For this review, take the finished solid that the model builds, in its own axes (mm). A direction names the side the tool comes from. Round coordinates to 2 decimals unless told otherwise and drop trailing zeros. Write each loop counter-clockwise with the first axis right and the second up, starting at its lowest first coordinate (ties: lowest second). Pieces come first, ordered by that corner, then holes. Notation, with made-up numbers: (-22, 88) - (19, 88) arc R17 cw to (19, 96) - close; hole circle Ø3 at (-31.75, 37). An arc over 180 degrees is marked (long way). Answer in a Markdown table with one row per item. Add a question column.
from build123d import *

# Parameters (mm, degrees)
SKETCH_1_R          = 29
EXTRUDE_1_DEPTH     = 6
SKETCH_2_R          = 12
EXTRUDE_2_DEPTH     = 20
SKETCH_3_R          = 2
CUT_EXTRUDE_1_DEPTH = 10
SKETCH_4_R          = 3
CUT_EXTRUDE_2_DEPTH = 30


with BuildPart() as part:
    # 草图1 → 凸台-拉伸1 (new body)
    with BuildSketch(Plane.XY):
        Circle(SKETCH_1_R)
    extrude(amount=EXTRUDE_1_DEPTH)

    # 草图2 → 凸台-拉伸2 (add)
    with BuildSketch(Plane.XY.offset(6)):
        Circle(SKETCH_2_R)
    extrude(amount=EXTRUDE_2_DEPTH)

    # 草图3 → 切除-拉伸1 (cut)
    with BuildSketch(Plane.XY.offset(6)):
        with Locations((0, 24)):
            Circle(SKETCH_3_R)
        with Locations((20.784609691, 12)):
            Circle(SKETCH_3_R)
        with Locations((20.784609691, -12)):
            Circle(SKETCH_3_R)
        with Locations((0, -24)):
            Circle(SKETCH_3_R)
        with Locations((-20.784609691, -12)):
            Circle(SKETCH_3_R)
        with Locations((-20.784609691, 12)):
            Circle(SKETCH_3_R)
    extrude(amount=-CUT_EXTRUDE_1_DEPTH, mode=Mode.SUBTRACT)

    # 草图4 → 切除-拉伸2 (cut)
    with BuildSketch(Plane.XY.offset(26)):
        Circle(SKETCH_4_R)
    extrude(amount=-CUT_EXTRUDE_2_DEPTH, mode=Mode.SUBTRACT)


solid = part.part
Q1. Insertion check: pin 1 Ø1 at (y, z) = (14.5, 5) entering from +X; pin 2 Ø7 at (x, y) = (0, 0) entering from +Z; pin 3 Ø2 at (x, z) = (7.5, 3.5) entering from -Y; pin 4 Ø3 at (x, y) = (-20.5, 15) entering from +Z. Each pin has a flat end and moves straight along its axis. Give the tip position at first contact, or say it passes through.
Q2. To check wall thickness, follow probe 1 along Y at (x, z) = (0, 18); probe 2 along Z at (x, y) = (-22.5, -17); probe 3 along Y at (x, z) = (-1, 15). State the ranges of each line that lie inside material, in increasing order.
Q3. Add section A-A on x = 0. State the section outline as (y, z) points, then the cut area to 3 significant figures.
Q4. Add section C-C on z = 16.5. State the section outline as (x, y) points, then the cut area to 3 significant figures.
Q5. Add section B-B on y = 0. State the section outline as (x, z) points, then the cut area to 3 significant figures.
Q6. Draft analysis for pull direction X (two halves, no side actions). For faces 1 (the face through (-3, 0, 13)), 2 (the face through (20.524, 13.983, 3.042)), 3 (the face through (12.5, 0.4, 6)), 4 (the face through (13.38, -25.73, 2.96)), state which applies: released by +X, released by -X, zero draft, split by the parting line, or undercut.
Q7. Add section D-D on x = 22. State the section outline as (y, z) points.
Q8. Tool access review of faces 5 (the face through (-11.99, 0.53, 15.86)), 6 (the face through (0.923, 22.226, 3.042)): name each direction out of +Z, -Z, +X, -X, +Y, -Y from which nothing blocks a thin tool from reaching the whole face with its end or side.
Answer sheet:
| question | item | result |
|---|---|---|
| 1 | pin 1 | stops at x = 25.4 |
| 1 | pin 2 | stops at z = 26 |
| 1 | pin 3 | stops at y = -28.26 |
| 1 | pin 4 | stops at z = 6 |
| 2 | probe 1 | y = -12 to -3, 3 to 12 |
| 2 | probe 2 | z = 0 to 6 |
| 2 | probe 3 | y = -11.96 to -2.83, 2.83 to 11.96 |
| 3 | outline | (-29, 0) - (-26, 0) - (-26, 6) - (-29, 6) - close; (-22, 0) - (-3, 0) - (-3, 26) - (-12, 26) - (-12, 6) - (-22, 6) - close; (3, 0) - (22, 0) - (22, 6) - (12, 6) - (12, 26) - (3, 26) - close; (26, 0) - (29, 0) - (29, 6) - (26, 6) - close |
| 3 | area | 624 mm² |
| 4 | outline | circle Ø24 at (0, 0); hole circle Ø6 at (0, 0) |
| 4 | area | 424 mm² |
| 5 | outline | (-29, 0) - (-3, 0) - (-3, 26) - (-12, 26) - (-12, 6) - (-29, 6) - close; (3, 0) - (29, 0) - (29, 6) - (12, 6) - (12, 26) - (3, 26) - close |
| 5 | area | 672 mm² |
| 6 | face 1 | undercut |
| 6 | face 2 | undercut |
| 6 | face 3 | zero draft |
| 6 | face 4 | split by the parting line |
| 7 | outline | (-18.89, 0) - (-13.59, 0) - (-13.59, 6) - (-18.89, 6) - close; (-10.41, 0) - (10.41, 0) - (10.41, 6) - (-10.41, 6) - close; (13.59, 0) - (18.89, 0) - (18.89, 6) - (13.59, 6) - close |
| 8 | face 5 | +Z |
| 8 | face 6 | +Z, -Z |
